Autodesk Inventor part; units mm, degrees
ref_plane "YZ Plane" through (0, 0, 0) normal (1, 0, 0) x (0, 1, 0)
ref_plane "XZ Plane" through (0, 0, 0) normal (0, 1, 0) x (-1, 0, 0)
ref_plane "XY Plane" through (0, 0, 0) normal (0, 0, 1) x (1, 0, 0)
sketch "Sketch1" plane through (0, 0, 0) normal (0, 1, 0) x (-1, 0, 0)
  line L0 (-0.8, 12.42) -> (0.8, 12.42)
  line L1 (0.8, 12.42) -> (0.8, 0)
  line L2 (0.8, 0) -> (-0.8, 0)
  line L3 (-0.8, 0) -> (-0.8, 12.42)
  line L4 (-0.8, 12.42) -> (0.8, 0) construction
  line L5 (0.8, 12.42) -> (-0.8, 0) construction
  line L6 (1.12, 0) -> (-1.12, 0)
  line L7 (0, -2.904) -> (0, 14.974)
  line L8 (-0.605, 0) -> (0.605, 0)
  line L9 (0.605, 0) -> (0.605, -0.35)
  line L10 (0.605, -0.35) -> (-0.605, -0.35)
  line L11 (-0.605, -0.35) -> (-0.605, 0)
  point P0 (0, 6.21)
  point P1 (-1.12, 0)
  point P2 (0, 6.21)
  dimension "d0" = 1.6
  dimension "d3" = 12.42
  dimension "d12" = 1.21
  dimension "d13" = 0.35
extrude "Extrusion1" add sketch "Sketch1" along normal blind 0.2
sketch "Sketch2" plane through (0.8, 0, 12.42) normal (1, 0, 0) x (0, 0, -1)
  line L0 (0, 0.2) -> (12.42, 0.2)
  line L1 (-0.1349, 0.2) -> (-0.4743, -0.64)
  line L2 (-0.4743, -0.64) -> (-0.2888, -0.7149)
  line L3 (-0.2888, -0.7149) -> (0, 0)
  line L4 (0, 0) -> (12.42, 0)
  line L5 (-0.1349, 0.2) -> (0, 0.2)
  line L6 (0, 0) -> (0, 0.2)
  line L7 (0, 0.2) -> (0, 0)
  dimension "d46" = 0.2
  dimension "d47" = 112
  dimension "d48" = 112
  dimension "d49" = 0.64
extrude "Extrusion2" add sketch "Sketch2" against normal up to surface (1.6 mm away)
sketch "Sketch3" plane through (0.8, -0.84, 14.02) normal (1, 0, 0) x (0, 0, -1)
  line L0 (14.02, 0.84) -> (1.6, 0.84)
  line L1 (-0.15, 0.2) -> (1.3414, 0.2)
  line L2 (1.3414, 0.2) -> (1.2606, 0)
  line L3 (1.2606, 0) -> (-0.15, 0)
  line L4 (-0.15, 0) -> (-0.15, 0.2)
  line L5 (1.3112, 0.1251) -> (1.6, 0.84)
  point P0 (1.1257, 0.2)
  dimension "d52" = 0.2
  dimension "d53" = 1.75
extrude "Extrusion3" add sketch "Sketch3" against normal up to surface (1.6 mm away)
sketch "Sketch4" plane through (0.605, 0, -0.35) normal (0, 0, -1) x (-1, 0, 0)
  line L0 (0, 0) -> (0, 0.2)
  line L1 (0, 0.2) -> (1.21, 0.2)
  line L2 (1.21, 0.2) -> (1.21, -3.495)
  line L3 (1.21, -3.495) -> (0, -3.495)
  line L4 (0, -3.495) -> (0, 0.2)
  line L5 (0.355, -3.495) -> (0.855, -3.495)
  line L6 (0.855, -3.495) -> (0.855, -7.81)
  line L7 (0.855, -7.81) -> (0.355, -7.81)
  line L8 (0.355, -7.81) -> (0.355, -3.495)
  line L9 (0, -3.495) -> (0.355, -3.85)
  line L10 (0, -3.495) -> (0.502, -3.495) construction
  line L11 (1.21, -3.495) -> (0.855, -3.85)
  line L12 (1.21, -3.495) -> (1.712, -3.495) construction
  line L13 (0.355, -7.477) -> (0.5184, -7.76)
  line L14 (0.6916, -7.76) -> (0.855, -7.477)
  arc A0 (0.5184, -7.76) -> (0.6916, -7.76) centre (0.605, -7.71) ccw
  line L15 (0.355, -7.477) -> (0.855, -7.477) construction
  point P0 (0.605, 0)
  dimension "d14" = 1.21
  dimension "d16" = 0.5
  dimension "d17" = 4.315
  dimension "d18" = 0.355
  dimension "d19" = 0.355
  dimension "d20" = 45
  dimension "d21" = 135
  dimension "d26" = 0.1
  dimension "d28" = 150
  dimension "d29" = 150
  dimension "d30" = 4.05
extrude "Extrusion4" add sketch "Sketch4" along normal blind 0.2 contours L0 L1 L2 L3 L4 | L3 L8 L9 | L3 L6 L14 A0 L13 L8 | L11 L6 L3
sketch "Sketch5" plane through (0, 0.2, 0) normal (0, 1, 0) x (1, 0, 0)
  line L0 (0.8, 0) -> (0.8, -12.42)
  line L1 (0.8, -1.6623) -> (0.605, -2)
  line L2 (-0.605, -2) -> (-0.8, -1.6623)
  line L3 (-0.8, 0) -> (-0.8, -12.5549)
  line L4 (0.8, -1.6623) -> (-0.8, -1.6623) construction
  line L5 (0.8, 0) -> (0.605, 0) construction
  line L6 (-0.605, 0) -> (-0.8, 0) construction
  line L7 (0.8, -1.6623) -> (0.8, -14.17)
  line L8 (-0.8, -14.17) -> (-0.8, -1.6623)
  line L9 (0.605, -2) -> (0.605, -14.17)
  line L10 (-0.605, -14.17) -> (-0.605, -2)
  line L11 (0.8, -14.17) -> (0.605, -14.17)
  line L12 (0, 3.504) -> (0, -17.174)
  line L13 (0.8, -14.17) -> (-0.8, -14.17)
  line L14 (-0.605, -14.17) -> (-0.8, -14.17)
  line L15 (-0.8, -12.8943) -> (-0.8, -14.17)
  point P0 (0, 0)
  point P1 (0.8, -12.62)
  point P2 (-0.8, -12.82)
  point P3 (-0.8, -12.62)
  dimension "d35" = 1.21
  dimension "d38" = 30
  dimension "d39" = 30
  dimension "d40" = 2
extrude "Extrusion5" cut sketch "Sketch5" against normal up to surface (1.04 mm away)
fillet "Fillet1" radius 0.3 1 edges at (0, 0, -0.35)
fillet "Fillet1" radius 0.5 1 edges at (0, 0.2, -0.55)
fillet "Fillet2" radius 0.3 2 edges at (0, 0.2, 12.5549) (0, -0.84, 12.7594)
fillet "Fillet2" radius 0.1 2 edges at (0, 0, 12.42) (0, -0.64, 12.8943)
equation "\"d48\" = d47"
equation "\"d18\" = d19"
equation "\"d39\" = d38"
equation "\"BendReliefWidth\" = Thickness"
equation "\"BendReliefDepth\" = 0.5 * Thickness"
equation "\"CornerReliefSize\" = 4 * Thickness"
equation "\"MinimumRemnant\" = 2 * Thickness"
equation "\"TransitionRadius\" = BendRadius"
equation "\"JacobiRadiusSize\" = BendRadius"
equation "\"GapSize\" = Thickness"
properties part number "USB 3.0 A Recepticle Upper Pin" material "Nickel-Copper Alloy 400"
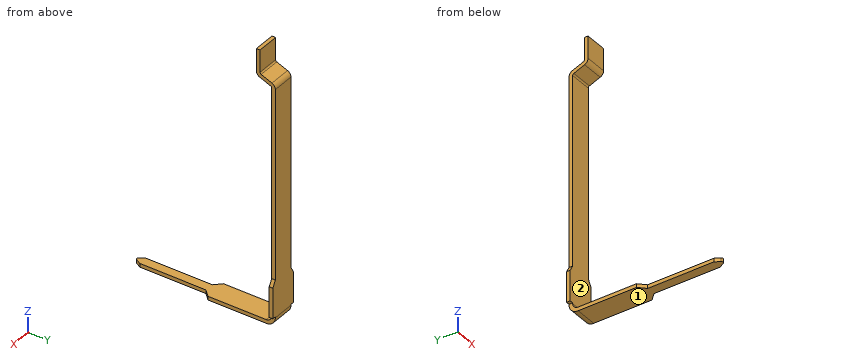
Design review of the part built by this model. Coordinates are the model's own, in mm. Face numbers are marked on the shaded views. A direction names the side the tool comes from. Round coordinates to 2 decimals unless told otherwise and drop trailing zeros. Order: outer loops, then holes, each group sorted by start corner. A loop starts at its lowest first (then second) coordinate and runs counter-clockwise, first axis right, second up. Notation, with made-up numbers: M 0.25,-0.5 L 41.25,-0.5 A22 ccw 41.25,17.5 Z; hole C -19,44 d6. An arc over 180 degrees is marked long. Put each result on its own line as item: value.
Q1. Machinability: for the marked faces 1 and 2, which of the approach directions +Z, -Z, +X, -X, +Y, -Y give a long, thin tool a straight path to every point of the face, cutting with its end or side? Answer none if there is none.
Reported:
face 1: -Z, +X, -X, +Y, -Y
face 2: +X, -X, -Y
Q2. Consider section A-A (z = 5.75). State the section outline as (x, y) points (3 decimals).
Reported:
outline: M -0.605,0 L 0.605,0 L 0.605,0.2 L -0.605,0.2 Z
Q3. Insertion check: pin 1 Ø1.1 at (y, z) = (-0.5, 9) entering from +X (3 decimals); pin 2 Ø0.5 at (x, z) = (0, 6) entering from -Y. Each pin has a flat end and moves straight along its axis. Give the tip position at first contact, or say it passes through.
Reported:
pin 1: x = 0.605
pin 2: y = 0
Q4. Consider section B-B (y = -6.75). State the section outline as (x, z) points.
Reported:
outline: M -0.25,-0.55 L 0.25,-0.55 L 0.25,-0.35 L -0.25,-0.35 Z
Q5. To check wall thickness, follow line 1 (Z direction, x = 0.1, y = -2.25); line 2 (Y direction, x = 0.55, z = 2.5); line 3 (Z direction, x = -0.45, y = -0.25). State the ranges of each line that lie inside material, in increasing order.
Reported:
line 1: -0.55 to -0.35
line 2: 0 to 0.2
line 3: -0.55 to -0.35, 12.52 to 12.74
